Can you work these out from the drawing? Everything is in mm from the part's minimum corner. A direction names the side the tool comes from. Round coordinates to 2 decimals unless told otherwise and drop trailing zeros. Loops run counter-clockwise (first coordinate to the right, second up) from the corner with the lowest first, then second, coordinate; pieces in that order, holes last. Notation, with made-up numbers: M -4,43.5 L 35,43.5 A14 ccw 35,53.5 Z; hole C -34,78 d9. An arc over 180 degrees is marked long. Use a Markdown table: item, result.
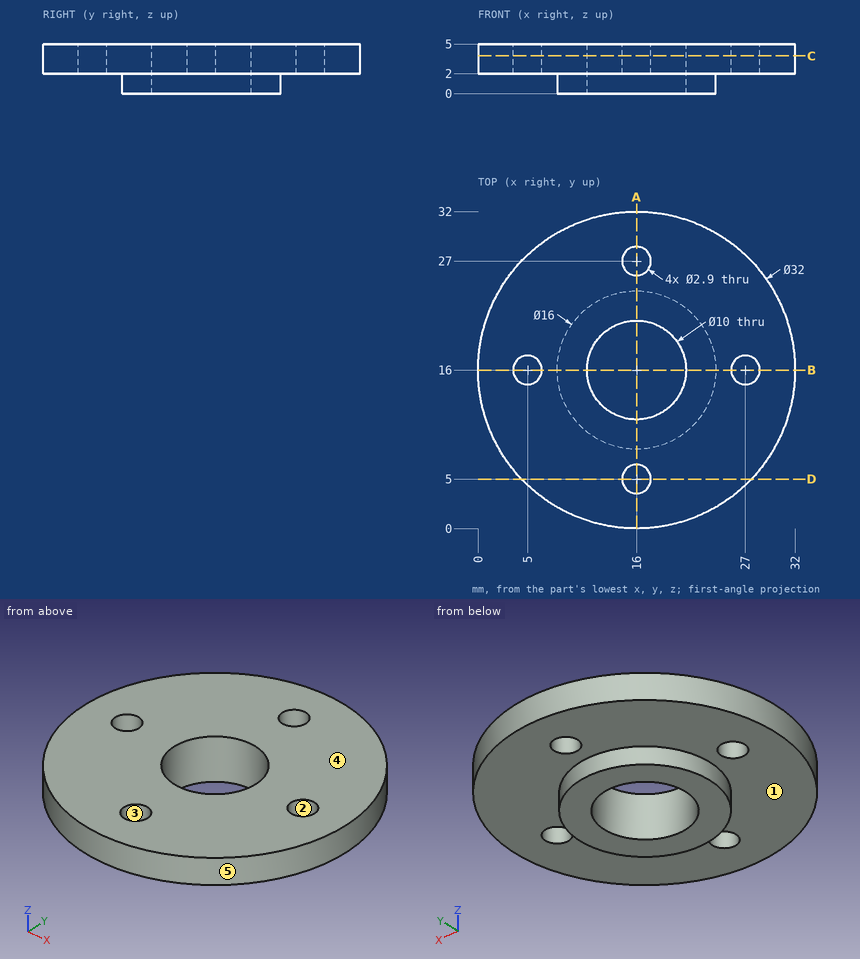
1. Imagine slicing it at C-C, the plane z = 3.8. Write out the boundary of the cut face in (x, y).
Answer sheet:
| item | result |
|---|---|
| outline | C 16,16 d32; hole C 5,16 d2.9; hole C 16,16 d10; hole C 16,5 d2.9; hole C 16,27 d2.9; hole C 27,16 d2.9 |
2. Which directions (+Z, -Z, +X, -X, +Y, -Y) give clear straight access to the entire face, cutting with the end or side of a thin tool? Please do the marked faces 1 and 2.
Answer sheet:
| item | result |
|---|---|
| face 1 | -Z |
| face 2 | +Z, -Z |
3. For pin 1 Ø2.5 at (x, y) = (5, 16) entering from -Z (3 decimals), with a flat end and sliding along its axis, tell me the tip position at first contact or that it passes through.
Answer sheet:
| item | result |
|---|---|
| pin 1 | through |
4. I need wall thicknesses on probe 1 along Y at (x, z) = (16, 3); probe 2 along Z at (x, y) = (26.5, 10.5); probe 3 along X at (y, z) = (26, 3.3). Which ranges of each line are inside material? Lowest first, please. Write a range as from..to.
Answer sheet:
| item | result |
|---|---|
| probe 1 | 0..3.55, 6.45..11, 21..25.55, 28.45..32 |
| probe 2 | 2..5 |
| probe 3 | 3.51..14.95, 17.05..28.49 |
5. Imagine slicing it at A-A, the plane x = 16. Write out the boundary of the cut face in (y, z), then the cut area to 3 significant figures.
Answer sheet:
| item | result |
|---|---|
| outline | M 0,2 L 3.55,2 L 3.55,5 L 0,5 Z; M 6.45,2 L 8,2 L 8,0 L 11,0 L 11,5 L 6.45,5 Z; M 21,0 L 24,0 L 24,2 L 25.55,2 L 25.55,5 L 21,5 Z; M 28.45,2 L 32,2 L 32,5 L 28.45,5 Z |
| area | 60.6 mm2 |
6. Imagine slicing it at D-D, the plane y = 5. Write out the boundary of the cut face in (x, z).
Answer sheet:
| item | result |
|---|---|
| outline | M 4.38,2 L 14.55,2 L 14.55,5 L 4.38,5 Z; M 17.45,2 L 27.62,2 L 27.62,5 L 17.45,5 Z |
7. We'd pull the mould along X, two halves only. Please class the marked faces 3, 4 and 5: +X half, -X half, draft (parallel to the pull), parting line (faces both ways), or undercut.
Answer sheet:
| item | result |
|---|---|
| face 3 | undercut |
| face 4 | draft |
| face 5 | parting line |
